Part model, mm, in its own coordinate system. A direction names the side the tool comes from. Give positions to 0.01 mm unless a question says otherwise; leave off trailing zeros. Write each loop counter-clockwise with the first axis right and the second up, starting at its lowest first coordinate (ties: lowest second). Pieces come first, ordered by that corner, then holes. Notation, with made-up numbers: (32.5, 64.25) - (40.5, 64.25) arc R34 ccw to (40.5, 102.25) - close; hole circle Ø11 at (-25.5, 83). An arc over 180 degrees is marked (long way). Answer as a JSON object with one key per item and string values. Group by question number.
```python
from build123d import *

# Parameters (mm, degrees)
SKETCH_1_R          = 1.6
EXTRUDE_1_DEPTH     = 4
SKETCH_2_W          = 60
SKETCH_2_H          = 5
EXTRUDE_2_DEPTH     = 31
SKETCH_8_R          = 1.6
CUT_EXTRUDE_1_DEPTH = 48.16990566
SKETCH_9_R          = 3
CUT_EXTRUDE_2_DEPTH = 3.2
FILLET_2_R          = 1


with BuildPart() as part:
    # 草图1 → 凸台-拉伸1 (new body)
    with BuildSketch(Plane.XY):
        Polygon((20, 0), (30, 0), (30, 15), (-30, 15), (-30, 0), (-20, 0), (-20, 10), (20, 10), align=None)
        with Locations((-25, 5)):
            Circle(SKETCH_1_R, mode=Mode.SUBTRACT)
        with Locations((25, 5)):
            Circle(SKETCH_1_R, mode=Mode.SUBTRACT)
    extrude(amount=EXTRUDE_1_DEPTH)

    # 草图2 → 凸台-拉伸2 (add)
    with BuildSketch(Plane.XY.offset(4)):
        with Locations((0, 12.5)):
            Rectangle(SKETCH_2_W, SKETCH_2_H)
    extrude(amount=EXTRUDE_2_DEPTH)

    # 草图8 → 切除-拉伸1 (cut, through all)
    with BuildSketch(Plane.XZ.offset(-10)):
        with Locations((-15.5, 4.25)):
            Circle(SKETCH_8_R)
        with Locations((-0.5, 13.75)):
            Circle(SKETCH_8_R)
        with Locations((0.5, 21.25)):
            Circle(SKETCH_8_R)
        with Locations((15.5, 30.75)):
            Circle(SKETCH_8_R)
    extrude(amount=-CUT_EXTRUDE_1_DEPTH, mode=Mode.SUBTRACT)

    # 草图9 → 切除-拉伸2 (cut)
    with BuildSketch(Plane.XZ.offset(-10)):
        with Locations((-15.5, 4.25)):
            Circle(SKETCH_9_R)
        with Locations((-0.5, 13.75)):
            Circle(SKETCH_9_R)
        with Locations((0.5, 21.25)):
            Circle(SKETCH_9_R)
        with Locations((15.5, 30.75)):
            Circle(SKETCH_9_R)
    extrude(amount=-CUT_EXTRUDE_2_DEPTH, mode=Mode.SUBTRACT)

    # 圆角2
    fillet_2_edges = [part.edges().sort_by_distance(p)[0] for p in [
        (0, 10, 0),
        (-20, 5, 0),
        (-30, 7.5, 0),
        (-30, 15, 17.5),
        (30, 15, 17.5),
        (20, 10, 2),
        (-20, 10, 2),
        (30, 5, 4),
        (-30, 5, 4),
        (-30, 10, 19.5),
        (30, 10, 19.5),
        (-30, 12.5, 35),
        (0, 10, 35),
        (30, 12.5, 35),
        (0, 15, 35),
        (0, 15, 0),
        (30, 7.5, 0),
        (20, 5, 0),
    ]]
    fillet(fillet_2_edges, radius=FILLET_2_R)


solid = part.part
```
1) Drill centre lines: line 1 along Z through (x, y) = (15.5, 13.95); line 2 along Z through (x, y) = (0.5, 11.95); line 3 along X through (y, z) = (3, 2). Where is each one in solid material? Low to high. Write a range as from..to.
2) Which spindle directions (+Z, -Z, +X, -X, +Y, -Y) get a long thin tool onto all of the face, cutting with end or side? Do faces 4 (the flat face through (-23, 5, 4)), 5 (the flat face through (-30, 12, 15)), 6 (the flat face through (2, 13.2, 20)), 7 (the flat face through (20, 5, 2)), 8 (the flat face through (0, 13, 35)). Say none if no direction does.
3) Drop flat-ended pins along their axis: P1, Ø7, axis at x = -15.5, z = 4.25, coming from the -Y side; P2, Ø5, axis at x = -15.5, z = 4.25, coming from the -Y side; P3, Ø1.9, axis at x = 15.5, z = 30.75, coming from the -Y side; P4, Ø5, axis at x = -25, y = 5, coming from the +Z side. Give the stop position or say it passes through.
4) Saw through at C-C (x = 15.5). List the corners of the cut face in (y, z), and give its area (3 significant figures).
5) Saw through at B-B (y = 5). List the corners of the cut face in (x, z).
6) Two-plate mould, pull along Z, no slides. Class faces 1 (the flat face through (23, 5, 4)), 2 (the flat face through (-25, 0, 2)), 3 (the cylindrical face through (-1.15, 11.58, 10.82)): +Z half, -Z half, draft (parallel to the pull), parting line (faces both ways), or undercut.
7) Saw through at A-A (z = 30.75). List the corners of the cut face in (x, y), and give its area (3 significant figures).
8) Saw through at D-D (x = -0.5). List the corners of the cut face in (y, z).
Checks:
{
 "1": {"line 1": "0..29.15, 32.35..35", "line 2": "0..10.92, 16.58..18.25, 24.25..35", "line 3": "-30..-20, 20..30"},
 "2": {"face 4": "+Z, +X, -X, -Y", "face 5": "+Z, -Z, -X, +Y, -Y", "face 6": "-Y", "face 7": "+Z, -Z, -Y", "face 8": "+Z, +X, -X, +Y, -Y"},
 "3": {"P1": "y = 10", "P2": "y = 13.2", "P3": "through", "P4": "z = 4"},
 "4": {"outline": "(10, 1) arc R1 ccw to (11, 0) - (14, 0) arc R1 ccw to (15, 1) - (15, 29.15) - (13.2, 29.15) - (13.2, 27.75) - (10, 27.75) - close; (10, 33.75) - (13.2, 33.75) - (13.2, 32.35) - (15, 32.35) - (15, 34) arc R1 ccw to (14, 35) - (11, 35) arc R1 ccw to (10, 34) - close", "area": "149 mm2"},
 "5": {"outline": "(-30, 1) arc R1 ccw to (-29, 0) - (-26.6, 0) - (-26.6, 4) - (-29, 4) arc R1 ccw to (-30, 3) - close; (-23.4, 0) - (-21, 0) arc R1 ccw to (-20, 1) - (-20, 4) - (-23.4, 4) - close; (20, 1) arc R1 ccw to (21, 0) - (23.4, 0) - (23.4, 4) - (20, 4) - close; (26.6, 0) - (29, 0) arc R1 ccw to (30, 1) - (30, 3) arc R1 ccw to (29, 4) - (26.6, 4) - close"},
 "6": {"face 1": "+Z half", "face 2": "draft", "face 3": "undercut"},
 "7": {"outline": "(-30, 11) arc R1 ccw to (-29, 10) - (12.5, 10) - (12.5, 13.2) - (13.9, 13.2) - (13.9, 15) - (-29, 15) arc R1 ccw to (-30, 14) - close; (17.1, 13.2) - (18.5, 13.2) - (18.5, 10) - (29, 10) arc R1 ccw to (30, 11) - (30, 14) arc R1 ccw to (29, 15) - (17.1, 15) - close", "area": "274 mm2"},
 "8": {"outline": "(10, 1) arc R1 ccw to (11, 0) - (14, 0) arc R1 ccw to (15, 1) - (15, 12.15) - (13.2, 12.15) - (13.2, 10.75) - (10, 10.75) - close; (10, 16.75) - (13.2, 16.75) - (13.2, 15.35) - (15, 15.35) - (15, 20) - (13.2, 20) - (13.2, 18.42) - (10, 18.42) - close; (10, 24.08) - (13.2, 24.08) - (13.2, 22.5) - (15, 22.5) - (15, 34) arc R1 ccw to (14, 35) - (11, 35) arc R1 ccw to (10, 34) - close"}
}
